CAD build for the part. Positions are in the model's coordinates, mm. A direction names the side the tool comes from. Give positions to 0.01 mm unless a question says otherwise; leave off trailing zeros. Loops run counter-clockwise (first coordinate to the right, second up) from the corner with the lowest first, then second, coordinate; pieces in that order, holes last. Notation, with made-up numbers: (22, -21) - (26, -21) arc R15 ccw to (26, 3) - close; hole circle Ø3 at (43, -10.5). An arc over 180 degrees is marked (long way). Return JSON: item names as keys, results as strings.
from build123d import *

# Parameters (mm, degrees)
SKETCH1_W           = 42
SKETCH1_H           = 42
BOSS_EXTRUDE1_DEPTH = 40.5
SKETCH2_R           = 11
BOSS_EXTRUDE2_DEPTH = 2
SKETCH3_R           = 2.5
BOSS_EXTRUDE3_DEPTH = 21
FILLET1_R           = 5
SKETCH4_R           = 1.5
CUT_EXTRUDE1_DEPTH  = 10
CUT_EXTRUDE2_START  = -17
CUT_EXTRUDE2_DEPTH  = 17


with BuildPart() as part:
    # Sketch1 → Boss-Extrude1 (new body)
    with BuildSketch(Plane.XY):
        Rectangle(SKETCH1_W, SKETCH1_H)
    extrude(amount=BOSS_EXTRUDE1_DEPTH)

    # Sketch2 → Boss-Extrude2 (add)
    with BuildSketch(Plane.XY.offset(40.5)):
        with Locations(Location((0, 0, 0), (0, 0, 180))):
            Circle(SKETCH2_R)
    extrude(amount=BOSS_EXTRUDE2_DEPTH)

    # Sketch3 → Boss-Extrude3 (add)
    with BuildSketch(Plane.XY.offset(42.5)):
        with Locations(Location((0, 0, 0), (0, 0, 180))):
            Circle(SKETCH3_R)
    extrude(amount=BOSS_EXTRUDE3_DEPTH)

    # Fillet1
    fillet1_edges = [part.edges().sort_by_distance(p)[0] for p in [
        (21, -21, 20.25),
        (-21, -21, 20.25),
        (-21, 21, 20.25),
        (21, 21, 20.25),
    ]]
    fillet(fillet1_edges, radius=FILLET1_R)

    # Sketch4 → Cut-Extrude1 (cut)
    with BuildSketch(Plane.XY.offset(40.5)):
        with Locations((15.556349186, 15.556349186)):
            Circle(SKETCH4_R)
        with Locations((-15.556349186, -15.556349186)):
            Circle(SKETCH4_R)
        with Locations((15.556349186, -15.556349186)):
            Circle(SKETCH4_R)
        with Locations((-15.556349186, 15.556349186)):
            Circle(SKETCH4_R)
    extrude(amount=-CUT_EXTRUDE1_DEPTH, mode=Mode.SUBTRACT)

    # Sketch5 → Cut-Extrude2 (cut)
    with BuildSketch(Plane.XY.offset(63.5).offset(CUT_EXTRUDE2_START)):
        with BuildLine():
            Line((-2.024666714, 1.466534929), (2.024666714, 1.466534929))
            ThreePointArc((2.024666714, 1.466534929), (0, 2.5), (-2.024666714, 1.466534929))
        make_face()
    extrude(amount=CUT_EXTRUDE2_DEPTH, mode=Mode.SUBTRACT)


solid = part.part
1. Cut at D-D, the plane y = 7.5. Write the cut outline in (x, z).
Values follow:
{"outline": "(-21, 0) - (21, 0) - (21, 40.5) - (8.05, 40.5) - (8.05, 42.5) - (-8.05, 42.5) - (-8.05, 40.5) - (-21, 40.5) - close"}
2. Drop flat-ended pins along their axis: P1, Ø5, axis at x = 9, y = 1.5, coming from the +Z side; P2, Ø4, axis at x = -15.5, y = -3, coming from the -Z side; P3, Ø1.5, axis at x = -15, y = -15, coming from the +Z side; P4, Ø2, axis at x = -0.5, z = 52, coming from the +Y side. Give the stop position or say it passes through.
Values follow:
{"P1": "stops at z = 42.5", "P2": "stops at z = 0", "P3": "stops at z = 40.5", "P4": "stops at y = 1.47"}
3. Cut at C-C, the plane x = -5. Write the cut outline in (y, z), plus the area to 3 significant figures.
Values follow:
{"outline": "(-21, 0) - (21, 0) - (21, 40.5) - (9.8, 40.5) - (9.8, 42.5) - (-9.8, 42.5) - (-9.8, 40.5) - (-21, 40.5) - close", "area": "1,740 mm²"}
4. Cut at B-B, the plane y = 0. Write the cut outline in (x, z).
Values follow:
{"outline": "(-21, 0) - (21, 0) - (21, 40.5) - (11, 40.5) - (11, 42.5) - (2.5, 42.5) - (2.5, 63.5) - (-2.5, 63.5) - (-2.5, 42.5) - (-11, 42.5) - (-11, 40.5) - (-21, 40.5) - close"}
5. Drill centre lines: probe 1 along Y at (x, z) = (15, 34.5); probe 2 along Z at (x, y) = (-8.5, 2); probe 3 along Z at (x, y) = (-18.5, 1.5). Where is each one in solid material? Low to high.
Values follow:
{"probe 1": "y = -21 to -16.95, -14.16 to 14.16, 16.95 to 21", "probe 2": "z = 0 to 42.5", "probe 3": "z = 0 to 40.5"}
6. Pull direction Y, two halves, no side cores. Call faces 4 (the face through (19, 20, 21)), 5 (the face through (-21, 0, 20)), 6 (the face through (16, -16, 30.5)), 7 (the face through (-1.34, -2.11, 52.85)): +Y half, -Y half, draft (parallel to the pull), parting line (faces both ways), or undercut.
Values follow:
{"face 4": "+Y half", "face 5": "draft", "face 6": "undercut", "face 7": "parting line"}
7. Cut at A-A, the plane x = 0. Write the cut outline in (y, z), plus the area to 3 significant figures.
Values follow:
{"outline": "(-21, 0) - (21, 0) - (21, 40.5) - (11, 40.5) - (11, 42.5) - (2.5, 42.5) - (2.5, 46.5) - (1.47, 46.5) - (1.47, 63.5) - (-2.5, 63.5) - (-2.5, 42.5) - (-11, 42.5) - (-11, 40.5) - (-21, 40.5) - close", "area": "1,830 mm²"}
8. Which spindle directions (+Z, -Z, +X, -X, +Y, -Y) get a long thin tool onto all of the face, cutting with end or side? Do faces 1 (the face through (14.45, 16.57, 35.57)), 2 (the face through (0, 1.467, 55)), 3 (the face through (-20, -19, 21)). Say none if no direction does.
Values follow:
{"face 1": "+Z", "face 2": "+Z, +X, -X, +Y", "face 3": "+Z, -Z, -X, -Y"}
